Can you work these out from the drawing? Everything is in mm from the part's minimum corner. Give positions to 0.01 mm unless a question says otherwise; leave off trailing zeros. Loops run counter-clockwise (first coordinate to the right, second up) from the corner with the lowest first, then second, coordinate; pieces in that order, holes last.
Q1. I need wall thicknesses on line 1 (Y direction, x = 6.35, z = 5); line 2 (Y direction, x = 6.35, z = 7.25); line 3 (X direction, y = 5, z = 7.5). Which ranges of each line are inside material? Lowest first, please.
Q2. We'd pull the mould along X, two halves only. Please class the marked faces 1, 2 and 3: +X half, -X half, draft (parallel to the pull), parting line (faces both ways), or undercut.
Q3. If we section it at D-D (z = 2.75): Please give me the cut outline in (x, y).
Q4. If we section it at C-C (z = 1.75): Please give me the cut outline in (x, y).
Q5. Will this pin go through, and if not, where does the flat tip stop? P1, Ø4, axis at x = 4, z = 1.5, coming from the -Y side.
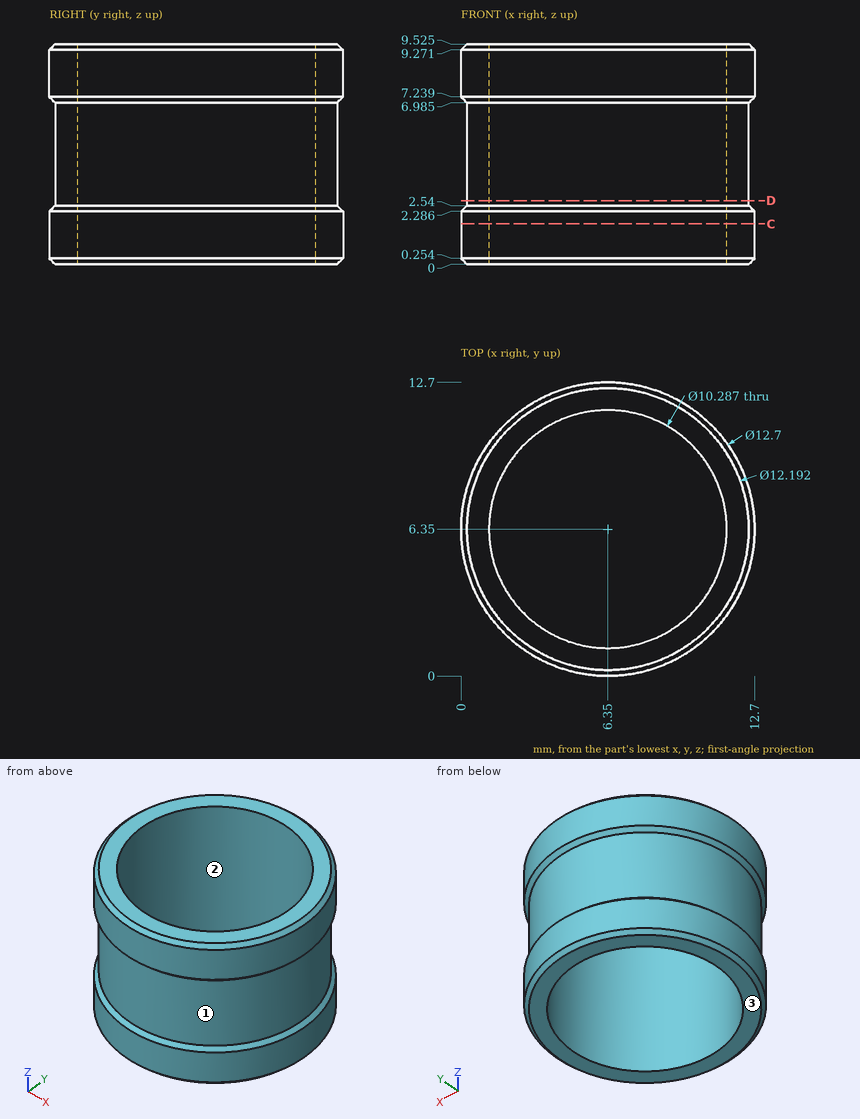
Check sheet entries:
1. line 1: y = 0.25 to 1.21, 11.49 to 12.45
1. line 2: y = 0 to 1.21, 11.49 to 12.7
1. line 3: x = 0.15 to 1.39, 11.31 to 12.55
2. face 1: parting line
2. face 2: undercut
2. face 3: draft
3. outline: circle Ø12.19 at (6.35, 6.35); hole circle Ø10.29 at (6.35, 6.35)
4. outline: circle Ø12.7 at (6.35, 6.35); hole circle Ø10.29 at (6.35, 6.35)
5. P1: stops at y = 0.01
